```python
from build123d import *

# Parameters (mm, degrees)
EXTRUDE_1_DEPTH         = 42.5
SKETCH_2_W              = 20
SKETCH_2_H              = 40.5
CUT_EXTRUDE_2_DEPTH     = 3
SKETCH_4_R              = 1.5
CUT_EXTRUDE_4_DEPTH     = 4
CUT_EXTRUDE_START       = -6
SKETCH_5_R              = 1.8
CUT_EXTRUDE_5_DEPTH     = 6
SKETCH_6_R              = 1.8
CUT_EXTRUDE_6_DEPTH     = 6
CUT_EXTRUDE_START_2     = -4
CUT_EXTRUDE_9_OUTLINE_R = 1.8
CUT_EXTRUDE_9_DEPTH     = 4
SKETCH_8_R              = 1.3
CUT_EXTRUDE_10_DEPTH    = 16
EXTRUDE_2_DEPTH         = 2
SKETCH_10_R             = 1.3
CUT_EXTRUDE_11_DEPTH    = 16


# Read off the part's stored shape, not the designer's step: 除料-伸長9
with BuildPart() as part:
    # 草圖1 → 填料-伸長1 (new body)
    with BuildSketch(Plane(origin=(0, 0, 0), x_dir=(1, 0, 0), z_dir=(0, 1, 0))):
        Polygon((36, 0), (61.1, 0), (61.1, -6), (-17.35, -6), (-17.35, 0), (0, 0), align=None)
    extrude(amount=EXTRUDE_1_DEPTH)

    # 草圖2 → 除料-伸長2 (cut)
    with BuildSketch(Plane.XY.offset(6)):
        with Locations((17, 21.25)):
            Rectangle(SKETCH_2_W, SKETCH_2_H)
    extrude(amount=-CUT_EXTRUDE_2_DEPTH, mode=Mode.SUBTRACT)

    # 草圖4 → 除料-伸長4 (cut)
    with BuildSketch(Plane.XY.offset(3)):
        with Locations((23.5, 29.25)):
            Circle(SKETCH_4_R)
        with Locations((10.5, 29.25)):
            Circle(SKETCH_4_R)
        with Locations((10.5, 13.25)):
            Circle(SKETCH_4_R)
        with Locations((23.5, 13.25)):
            Circle(SKETCH_4_R)
    extrude(amount=-CUT_EXTRUDE_4_DEPTH, mode=Mode.SUBTRACT)

    # 草圖5 → 除料-伸長5 (cut)
    with BuildSketch(Plane(origin=(0, 0, 0), x_dir=(-1, 0, 0), z_dir=(0, 0, -1)).offset(CUT_EXTRUDE_START)):
        with Locations((12.1, 29.25)):
            Circle(SKETCH_5_R)
        with Locations((12.1, 21.25)):
            Circle(SKETCH_5_R)
        with Locations((12.1, 13.25)):
            Circle(SKETCH_5_R)
    extrude(amount=CUT_EXTRUDE_5_DEPTH, mode=Mode.SUBTRACT)

    # 草圖6 → 除料-伸長6 (cut)
    with BuildSketch(Plane(origin=(0, 0, 0), x_dir=(-1, 0, 0), z_dir=(0, 0, -1)).offset(CUT_EXTRUDE_START)):
        with Locations((-57.1, 29.25)):
            Circle(SKETCH_6_R)
        with Locations((-57.1, 21.25)):
            Circle(SKETCH_6_R)
        with Locations((-57.1, 13.25)):
            Circle(SKETCH_6_R)
    extrude(amount=CUT_EXTRUDE_6_DEPTH, mode=Mode.SUBTRACT)

    # 除料-伸長9 outline → 除料-伸長9 (cut)
    # profile 1 of 2: a face of its own
    with BuildSketch(Plane(origin=(0, 0, 0), x_dir=(-1, 0, 0), z_dir=(0, 0, -1)).offset(CUT_EXTRUDE_START_2)):
        with BuildLine():
            Line((-60.95, 29.25), (-60.95, 13.25))
            ThreePointArc((-60.95, 13.25), (-57.1, 9.4), (-53.25, 13.25))
            Line((-53.25, 13.25), (-53.25, 29.25))
            ThreePointArc((-53.25, 29.25), (-57.1, 33.1), (-60.95, 29.25))
        make_face()
        with Locations((-57.1, 13.25)):
            Circle(CUT_EXTRUDE_9_OUTLINE_R, mode=Mode.SUBTRACT)
        with Locations((-57.1, 21.25)):
            Circle(CUT_EXTRUDE_9_OUTLINE_R, mode=Mode.SUBTRACT)
        with Locations((-57.1, 29.25)):
            Circle(CUT_EXTRUDE_9_OUTLINE_R, mode=Mode.SUBTRACT)
    # profile 2 of 2: a face of its own
    with BuildSketch(Plane(origin=(0, 0, 0), x_dir=(-1, 0, 0), z_dir=(0, 0, -1)).offset(CUT_EXTRUDE_START_2)):
        with BuildLine():
            Line((8.1, 21.25), (8.155316246, 12.587074601))
            ThreePointArc((8.155316246, 12.587074601), (12.1, 9.25), (16.044683754, 12.587074601))
            Line((16.044683754, 12.587074601), (16.1, 21.25))
            Line((16.1, 21.25), (16.1, 29.25))
            ThreePointArc((16.1, 29.25), (12.1, 33.25), (8.1, 29.25))
            Line((8.1, 29.25), (8.1, 21.25))
        make_face()
        with Locations((12.1, 13.25)):
            Circle(CUT_EXTRUDE_9_OUTLINE_R, mode=Mode.SUBTRACT)
        with Locations((12.1, 21.25)):
            Circle(CUT_EXTRUDE_9_OUTLINE_R, mode=Mode.SUBTRACT)
        with Locations((12.1, 29.25)):
            Circle(CUT_EXTRUDE_9_OUTLINE_R, mode=Mode.SUBTRACT)
    extrude(amount=CUT_EXTRUDE_9_DEPTH, mode=Mode.SUBTRACT)

    # 草圖8 → 除料-伸長10 (cut)
    with BuildSketch(Plane(origin=(0, 0, 0), x_dir=(-1, 0, 0), z_dir=(0, 0, -1))):
        with Locations((-4, 31.25)):
            Circle(SKETCH_8_R)
        with Locations((-4, 21.25)):
            Circle(SKETCH_8_R)
        with Locations((-4, 11.25)):
            Circle(SKETCH_8_R)
        with Locations((-30, 11.25)):
            Circle(SKETCH_8_R)
        with Locations((-30, 21.25)):
            Circle(SKETCH_8_R)
        with Locations((-30, 31.25)):
            Circle(SKETCH_8_R)
    extrude(amount=-CUT_EXTRUDE_10_DEPTH, mode=Mode.SUBTRACT)

    # 草圖9 → 填料-伸長2 (add)
    with BuildSketch(Plane.XY.offset(6)):
        Polygon((7, 41.5), (7, 42.5), (2, 42.5), (2, 0), (7, 0), (7, 1), align=None)
        Polygon((27, 41.5), (27, 42.5), (33, 42.5), (33, 0), (27, 0), align=None)
    extrude(amount=EXTRUDE_2_DEPTH)

    # 草圖10 → 除料-伸長11 (cut)
    with BuildSketch(Plane(origin=(0, 0, 0), x_dir=(-1, 0, 0), z_dir=(0, 0, -1))):
        with Locations((-30, 31.25)):
            Circle(SKETCH_10_R)
        with Locations((-30, 21.25)):
            Circle(SKETCH_10_R)
        with Locations((-30, 11.25)):
            Circle(SKETCH_10_R)
        with Locations((-4, 11.25)):
            Circle(SKETCH_10_R)
        with Locations((-4, 21.25)):
            Circle(SKETCH_10_R)
        with Locations((-4, 31.25)):
            Circle(SKETCH_10_R)
    extrude(amount=-CUT_EXTRUDE_11_DEPTH, mode=Mode.SUBTRACT)


solid = part.part
```
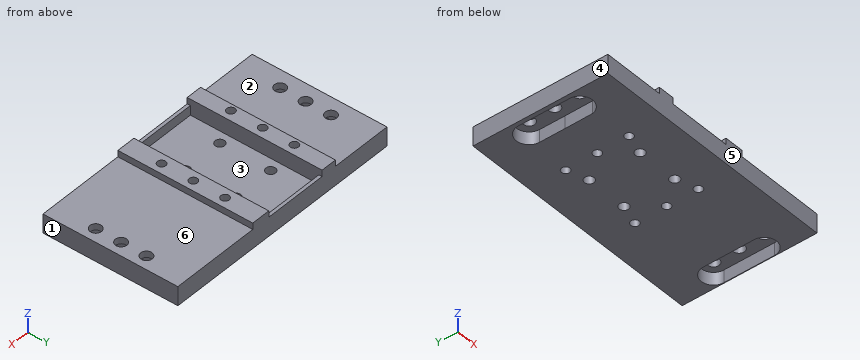
Work out the finished part from the listing and answer in its coordinate system (mm). Face numbers are marked on the shaded views. A direction names the side the tool comes from. Coordinates: 2 decimals unless noted, no trailing zeros. Write each loop counter-clockwise with the first axis right and the second up, starting at its lowest first coordinate (ties: lowest second). Pieces come first, ordered by that corner, then holes.
Q1. A cutting plane is placed at B-B, the plane z = 2.25. State how many separate pieces and enclosed holes the cut face has, then the cut area to 3 significant figures.
Q2. Determine the mould class of the marked faces 1, 2, 3 and 4 for opening direction X: released by +X, released by -X, zero draft, split by the parting line, or undercut.
Q3. A cutting plane is placed at D-D, the plane y = 36. Give the vertices of the cut face in (x, z).
Q4. A cutting plane is placed at C-C, the plane x = 57.1. Give the vertices of the cut face in (y, z), then the cut area to 3 significant figures.
Q5. A cutting plane is placed at A-A, the plane x = 10.5. Give the vertices of the cut face in (y, z).
Q6. Which of the six approach directions +Z, -Z, +X, -X, +Y, -Y give full straight-line access (tool end or side, diameter ignored) to the marked faces 5 and 6?
Q7. Each of these flat-tipped pins is pushed along its axis until it touches: pin 1 Ø3.5 at (x, y) = (30, 31.25) entering from -Z; pin 2 Ø4.5 at (x, y) = (-12.1, 13.25) entering from +Z; pin 3 Ø2.5 at (x, y) = (10.5, 29.25) entering from -Z; pin 4 Ø4 at (x, y) = (23.5, 13.25) entering from +Z. Where does it stop, or does it pass through?
Q8. Find the intervals of material crossed by line 1 (Y direction, x = 4, z = 3.75); line 2 (Y direction, x = 57.1, z = 4.75); line 3 (Y direction, x = 16, z = 3.5), in increasing order.
Findings below:
1. separate pieces: 1
1. enclosed holes: 12
1. area: 2,930 mm2
2. face 1: released by +X
2. face 2: zero draft
2. face 3: undercut
2. face 4: released by -X
3. outline: (-17.35, 0) - (61.1, 0) - (61.1, 6) - (33, 6) - (33, 8) - (27, 8) - (27, 3) - (7, 3) - (7, 8) - (2, 8) - (2, 6) - (-17.35, 6) - close
4. outline: (0, 0) - (9.4, 0) - (9.4, 4) - (11.45, 4) - (11.45, 6) - (0, 6) - close; (15.05, 4) - (19.45, 4) - (19.45, 6) - (15.05, 6) - close; (23.05, 4) - (27.45, 4) - (27.45, 6) - (23.05, 6) - close; (31.05, 4) - (33.1, 4) - (33.1, 0) - (42.5, 0) - (42.5, 6) - (31.05, 6) - close
4. area: 139 mm2
5. outline: (0, 0) - (11.75, 0) - (11.75, 3) - (1, 3) - (1, 6) - (0, 6) - close; (14.75, 0) - (27.75, 0) - (27.75, 3) - (14.75, 3) - close; (30.75, 0) - (42.5, 0) - (42.5, 6) - (41.5, 6) - (41.5, 3) - (30.75, 3) - close
6. face 5: +Z, -Z, +X, -X, -Y
6. face 6: +Z, +X, +Y, -Y
7. pin 1: stops at z = 0
7. pin 2: stops at z = 6
7. pin 3: passes through
7. pin 4: stops at z = 3
8. line 1: y = 0 to 9.95, 12.55 to 19.95, 22.55 to 29.95, 32.55 to 42.5
8. line 2: y = 0 to 11.45, 15.05 to 19.45, 23.05 to 27.45, 31.05 to 42.5
8. line 3: y = 0 to 1, 41.5 to 42.5
